from build123d import *

# Parameters (mm, degrees)
SKETCH1_W           = 250
SKETCH1_H           = 150
BOSS_EXTRUDE1_DEPTH = 114
SKETCH4_W           = 158.825989779
SKETCH4_H           = 169.09880145
CUT_EXTRUDE1_DEPTH  = 114
SKETCH5_R           = 21.25669472
CUT_EXTRUDE2_DEPTH  = 54


with BuildPart() as part:
    # Sketch1 → Boss-Extrude1 (new body)
    with BuildSketch(Plane.XY):
        Rectangle(SKETCH1_W, SKETCH1_H)
    extrude(amount=BOSS_EXTRUDE1_DEPTH)

    # Sketch4 → Cut-Extrude1 (cut)
    with BuildSketch(Plane(origin=(27.906934923, -24.538252492, -40.49320945), x_dir=(0.8614948455361232, 0.2631519435385569, 0.4342553231988889), z_dir=(-0.5077663154588844, 0.4464731827403718, 0.7367734156299286))):
        with Locations((63.082324951, -59.282681283)):
            Rectangle(SKETCH4_W, SKETCH4_H)
    extrude(amount=-CUT_EXTRUDE1_DEPTH, mode=Mode.SUBTRACT)

    # Sketch5 → Cut-Extrude2 (cut)
    with BuildSketch(Plane(origin=(0, 0, 0), x_dir=(-1, 0, 0), z_dir=(0, 0, -1))):
        with Locations((25.521911399, 0)):
            Circle(SKETCH5_R)
    extrude(amount=-CUT_EXTRUDE2_DEPTH, mode=Mode.SUBTRACT)


solid = part.part
For this review, take the finished solid that the model builds, in its own axes (mm). A direction names the side the tool comes from. Round coordinates to 2 decimals unless told otherwise and drop trailing zeros. Write each loop counter-clockwise with the first axis right and the second up, starting at its lowest first coordinate (ties: lowest second). Pieces come first, ordered by that corner, then holes. Notation, with made-up numbers: (-39.5, 27.25) - (7.5, 27.25) arc R19 ccw to (7.5, 50.25) - close; hole circle Ø7 at (-17, -36). An arc over 180 degrees is marked (long way). Write item = value, one per line. Start each with the question number.
1. For faces 4 (the face through (125, -1, 69)), 5 (the face through (-25, 0, 54)), list the 3-axis set-ups (+Z, -Z, +X, -X, +Y, -Y) from which the entire face can be reached by the end or side of a thin tool; tool diameter is ignored.
2. Draft analysis for pull direction X (two halves, no side actions). For faces 1 (the face through (-4.286, 0.935, 26.622)), 2 (the face through (-125, -1, 56)), 3 (the face through (101.447, -44.957, 22.562)), state which applies: released by +X, released by -X, zero draft, split by the parting line, or undercut.
3. Consider section C-C on z = 35. State the section outline as (x, y) points, plus the area to 3 significant figures.
4. Consider section B-B on y = 15.5. State the section outline as (x, z) points, plus the area to 3 significant figures.
5. Consider section A-A on x = -8.5. State the section outline as (y, z) points, plus the area to 3 significant figures.
6. Consider section D-D on x = 95. State the section outline as (y, z) points, plus the area to 3 significant figures.
7. Wall thickness on L1, parallel to Y at x = -24, z = 33.5; L2, parallel to Y at x = -18, z = 11.5; L3, parallel to Z at x = -18.5, y = -7: over which ranges is each line inside the solid? List them lowest first.
Evaluation:
q1.face_4 = +Z, -Z, +X, +Y, -Y
q1.face_5 = -Z
q2.face_1 = undercut
q2.face_2 = released by -X
q2.face_3 = released by +X
q3.outline = (-125, -75) - (93.08, -75) - (125, -38.7) - (125, 75) - (-125, 75) - close; hole circle Ø42.51 at (-25.52, 0)
q3.area = 35,500 mm2
q4.outline = (-125, 0) - (-40.07, 0) - (-40.07, 54) - (-10.98, 54) - (-10.98, 0) - (121.87, 0) - (125, 2.16) - (125, 114) - (-125, 114) - close
q4.area = 26,900 mm2
q5.outline = (-75, 0) - (-12.73, 0) - (-12.73, 54) - (12.73, 54) - (12.73, 0) - (75, 0) - (75, 114) - (-75, 114) - close
q5.area = 15,700 mm2
q6.outline = (-75, 36.32) - (-15.06, 0) - (75, 0) - (75, 114) - (-75, 114) - close
q6.area = 16,000 mm2
q7.L1 = -75 to -21.2, 21.2 to 75
q7.L2 = -75 to -19.88, 19.88 to 75
q7.L3 = 54 to 114
